```python
from build123d import *

# Parameters (mm, degrees)
F0_W     = 120
F0_H     = 45
F1_DEPTH = 3
F2_W     = 120
F2_H     = 45
F2_W_2   = 114
F2_H_2   = 26
F3_DEPTH = 20
F5_W     = 120
F5_H     = 2
F6_DEPTH = 17
F7_DEPTH = 13


with BuildPart() as f1:
    # F0 (on Top) → F1 (new body)
    with BuildSketch(Plane.XY):
        Rectangle(F0_W, F0_H)
    extrude(amount=F1_DEPTH)

    # F2 (on face) → F3 (join)
    with BuildSketch(Plane.XY.offset(3)):
        Rectangle(F2_W, F2_H)
        with Locations((0, -6.5)):
            Rectangle(F2_W_2, F2_H_2, mode=Mode.SUBTRACT)
    extrude(amount=F3_DEPTH)

    # F5 (on face) → F6 (cut)
    with BuildSketch(Plane(origin=(0, 0, 0), x_dir=(1, 0, 0), z_dir=(0, 0, -1))):
        with Locations((0, -18.5)):
            Rectangle(F5_W, F5_H)
    extrude(amount=-F6_DEPTH, mode=Mode.SUBTRACT)

    # F4 (on face) → F7 (cut)
    with BuildSketch(Plane.XY.offset(23)):
        Polygon((-53, 8.035898), (-51, 11.5), (-53, 14.964102), (-57, 14.964102), (-59, 11.5), (-57, 8.035898), align=None)
        Polygon((-43, 8.035898), (-41, 11.5), (-43, 14.964102), (-47, 14.964102), (-49, 11.5), (-47, 8.035898), align=None)
        Polygon((-33, 8.035898), (-31, 11.5), (-33, 14.964102), (-37, 14.964102), (-39, 11.5), (-37, 8.035898), align=None)
        Polygon((-23, 8.035898), (-21, 11.5), (-23, 14.964102), (-27, 14.964102), (-29, 11.5), (-27, 8.035898), align=None)
        Polygon((-13, 8.035898), (-11, 11.5), (-13, 14.964102), (-17, 14.964102), (-19, 11.5), (-17, 8.035898), align=None)
        Polygon((-3, 8.035898), (-1, 11.5), (-3, 14.964102), (-7, 14.964102), (-9, 11.5), (-7, 8.035898), align=None)
        Polygon((3, 8.035898), (7, 8.035898), (9, 11.5), (7, 14.964102), (3, 14.964102), (1, 11.5), align=None)
        Polygon((11, 11.5), (13, 8.035898), (17, 8.035898), (19, 11.5), (17, 14.964102), (13, 14.964102), align=None)
        Polygon((29, 11.5), (27, 14.964102), (23, 14.964102), (21, 11.5), (23, 8.035898), (27, 8.035898), align=None)
        Polygon((33, 8.035898), (37, 8.035898), (39, 11.5), (37, 14.964102), (33, 14.964102), (31, 11.5), align=None)
        Polygon((43, 8.035898), (47, 8.035898), (49, 11.5), (47, 14.964102), (43, 14.964102), (41, 11.5), align=None)
        Polygon((57, 8.035898), (59, 11.5), (57, 14.964102), (53, 14.964102), (51, 11.5), (53, 8.035898), align=None)
    extrude(amount=-F7_DEPTH, mode=Mode.SUBTRACT)


solid = f1.part
```
Geometry: final body of the model. Coordinates: model frame, mm. Coordinates: 2 decimals unless noted, no trailing zeros. Write each loop counter-clockwise with the first axis right and the second up, starting at its lowest first coordinate (ties: lowest second). Pieces come first, ordered by that corner, then holes. Notation, with made-up numbers: M 87,68 L 145,68 A14 cw 145,88 Z; hole C 50,25 d3. An arc over 180 degrees is marked long. Use CSV: the item, a comma, the result in double quotes. Start each with the question number.
1. Cut plane A-A on z = 5. Return the cut outline in (x, y), plus the area to 3 significant figures.
2. Cut plane D-D on z = 14.5. Count the separate pieces of the cut face and the enclosed holes in it, plus the area to 3 significant figures.
3. First-contact query: P1, Ø2, axis at x = -25, y = 13, coming from the +Z side; P2, Ø8, axis at x = 15, y = -7.5, coming from the +Z side. Flat tips, straight axial feed; report the tip coordinate or a pass-through.
4. Cut plane C-C on y = -15.5. Return the cut outline in (x, z), plus the area to 3 significant figures.
5. Mould query, pull axis X, two halves, no side actions, for faces 1 (the face through (-42.014, 9.744, 16.591)), 2 (the face through (-60, 0, 11)), 3 (the face through (-45, 14.964, 17)). Classes: pulls with the +X half, pulls with the -X half, needs draft (parallel to the pull), parting line crosses it, or undercut.
6. Ray query, probe 1 along Y at (x, z) = (-1, 6.5); probe 2 along Y at (x, z) = (-36.5, 18.5); probe 3 along Y at (x, z) = (-25.5, 10.5). Return the intervals inside material, ascending.
7. Cut plane B-B on x = -35. Return the cut outline in (y, z).
Entries:
1,outline,"M -60,-22.5 L 60,-22.5 L 60,17.5 L -60,17.5 Z; M -60,19.5 L 60,19.5 L 60,22.5 L -60,22.5 Z; hole M -57,-19.5 L 57,-19.5 L 57,6.5 L -57,6.5 Z"
1,area,"2,200 mm²"
2,separate pieces,"2"
2,enclosed holes,"13"
2,area,"1,700 mm²"
3,P1,"z = 10"
3,P2,"z = 3"
4,outline,"M -60,0 L 60,0 L 60,23 L 57,23 L 57,3 L -57,3 L -57,23 L -60,23 Z"
4,area,"480 mm²"
5,face 1,"undercut"
5,face 2,"pulls with the -X half"
5,face 3,"undercut"
6,probe 1,"-22.5 to -19.5, 6.5 to 17.5, 19.5 to 22.5"
6,probe 2,"-22.5 to -19.5, 6.5 to 8.04, 14.96 to 22.5"
6,probe 3,"-22.5 to -19.5, 6.5 to 8.04, 14.96 to 17.5, 19.5 to 22.5"
7,outline,"M -22.5,0 L 17.5,0 L 17.5,17 L 19.5,17 L 19.5,0 L 22.5,0 L 22.5,23 L 14.96,23 L 14.96,10 L 8.04,10 L 8.04,23 L 6.5,23 L 6.5,3 L -19.5,3 L -19.5,23 L -22.5,23 Z"
